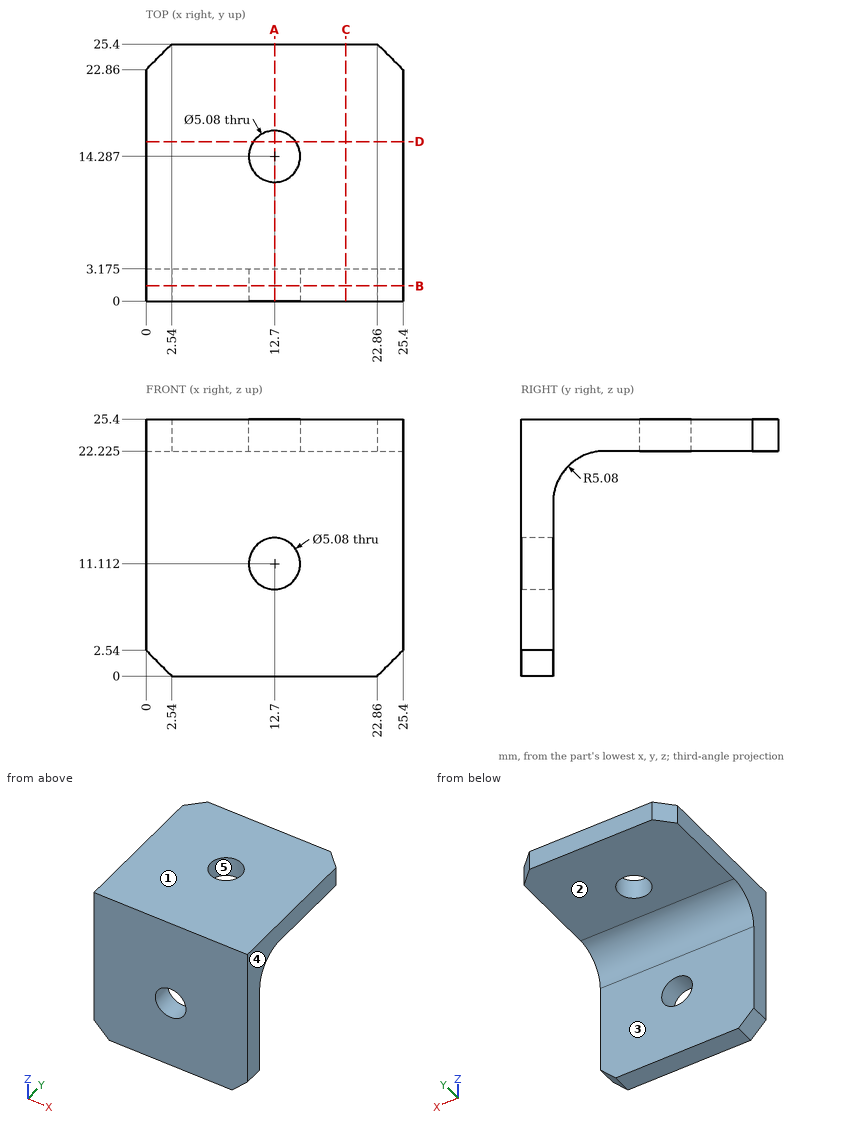
Geometry: see drawing. Coordinates: mm, zero at the bounding-box minimum. A direction names the side the tool comes from. Give positions to 0.01 mm unless a question says otherwise; leave off trailing zeros. Loops run counter-clockwise (first coordinate to the right, second up) from the corner with the lowest first, then second, coordinate; pieces in that order, holes last. Notation, with made-up numbers: (88.25, 42) - (146.25, 42) arc R17 cw to (146.25, 52) - close; hole circle Ø2 at (-8.5, 5.5). An arc over 180 degrees is marked (long way). Use CSV: the item, a comma, the result in double quotes. Start each with the question number.
1. Section C-C (x = 19.75). Output: boundary loops of the cut face in (y, z) (1 decimal), then the cut area to 3 significant figures.
2. Section B-B (y = 1.5). Output: boundary loops of the cut face in (x, z).
3. Ray query, L1, parallel to Y at x = 12.7, z = 23.8; L2, parallel to Y at x = 5.5, z = 8.5 (1 decimal); L3, parallel to Z at x = 15, y = 11.5 (1 decimal). Return the intervals inside material, ascending.
4. Reachability of the marked faces 1 and 2 from +Z, -Z, +X, -X, +Y, -Y: full face, straight path, thin tool, end or side. Return the list, or none.
5. Draft query along X for the marked faces 3, 4 and 5. Return one class per face: +X half, -X half, draft (parallel to the pull), parting line (faces both ways), or undercut.
6. Section A-A (x = 12.7). Output: boundary loops of the cut face in (y, z) (1 decimal).
7. Pin query (flat end, axial travel): pin 1 (5 mm diameter, centred on x = 12.5, y = 15.5, fed in from -Z) (1 decimal); pin 2 (2 mm diameter, centred on x = 11, z = 20, fed in from +Y) (1 decimal). Return the tip coordinate at first contact, or that it passes through.
8. Section D-D (y = 15.75). Output: boundary loops of the cut face in (x, z) (1 decimal).
Response:
1,outline,"(0, 0) - (3.2, 0) - (3.2, 17.1) arc R5.1 cw to (8.3, 22.2) - (25.4, 22.2) - (25.4, 25.4) - (0, 25.4) - close"
1,area,"157 mm²"
2,outline,"(0, 2.54) - (2.54, 0) - (22.86, 0) - (25.4, 2.54) - (25.4, 25.4) - (0, 25.4) - close; hole circle Ø5.08 at (12.7, 11.11)"
3,L1,"0 to 11.75, 16.83 to 25.4"
3,L2,"0 to 3.2"
3,L3,"22.2 to 25.4"
4,face 1,"+Z, +X, -X, +Y, -Y"
4,face 2,"-Z, +X, -X, +Y"
5,face 3,"draft"
5,face 4,"+X half"
5,face 5,"undercut"
6,outline,"(0, 0) - (3.2, 0) - (3.2, 8.6) - (0, 8.6) - close; (0, 13.7) - (3.2, 13.7) - (3.2, 17.1) arc R5.1 cw to (8.3, 22.2) - (11.7, 22.2) - (11.7, 25.4) - (0, 25.4) - close; (16.8, 22.2) - (25.4, 22.2) - (25.4, 25.4) - (16.8, 25.4) - close"
7,pin 1,"z = 22.2"
7,pin 2,"y = 4.9"
8,outline,"(0, 22.2) - (10.6, 22.2) - (10.6, 25.4) - (0, 25.4) - close; (14.8, 22.2) - (25.4, 22.2) - (25.4, 25.4) - (14.8, 25.4) - close"
